Check sheet for the drawn part. Datum: minimum x, y, z corner. Units: mm. Coordinates: 2 decimals unless noted, no trailing zeros. Loops run counter-clockwise (first coordinate to the right, second up) from the corner with the lowest first, then second, coordinate; pieces in that order, holes last. Notation, with made-up numbers: (46.25, 24.5) - (63.25, 24.5) arc R13 ccw to (63.25, 40.5) - close; hole circle Ø1 at (70, -7). An arc over 180 degrees is marked (long way). Answer as CSV lines item,"result". Start each with the question number.
1. Cross-section at A-A (x = 6). Enter the section's corners in (y, z).
2. Material ranges on line 1 (X direction, y = 1, z = 35); line 2 (Y direction, x = 3, z = 30); line 3 (X direction, y = 3.2, z = 2), recorded low to high. Write a range as [from, to].
3. Cross-section at B-B (z = 30). Enter the section's corners in (x, y).
4. Cross-section at D-D (y = 2.5). State how many separate pieces and enclosed holes the cut face has, plus the area to 3 significant figures.
5. Gauge pin test, flat ends, axial feed: P1, Ø2, axis at y = 2.5, z = 10, coming from the +X side; P2, Ø2, axis at x = 10, y = 2.5, coming from the -Z side; P3, Ø0.8, axis at y = 2, z = 10.5, coming from the -X side. Record the tip position at first contact, or that the pin passes through.
6. Cross-section at C-C (x = 37). Enter the section's corners in (y, z), plus the area to 3 significant figures.
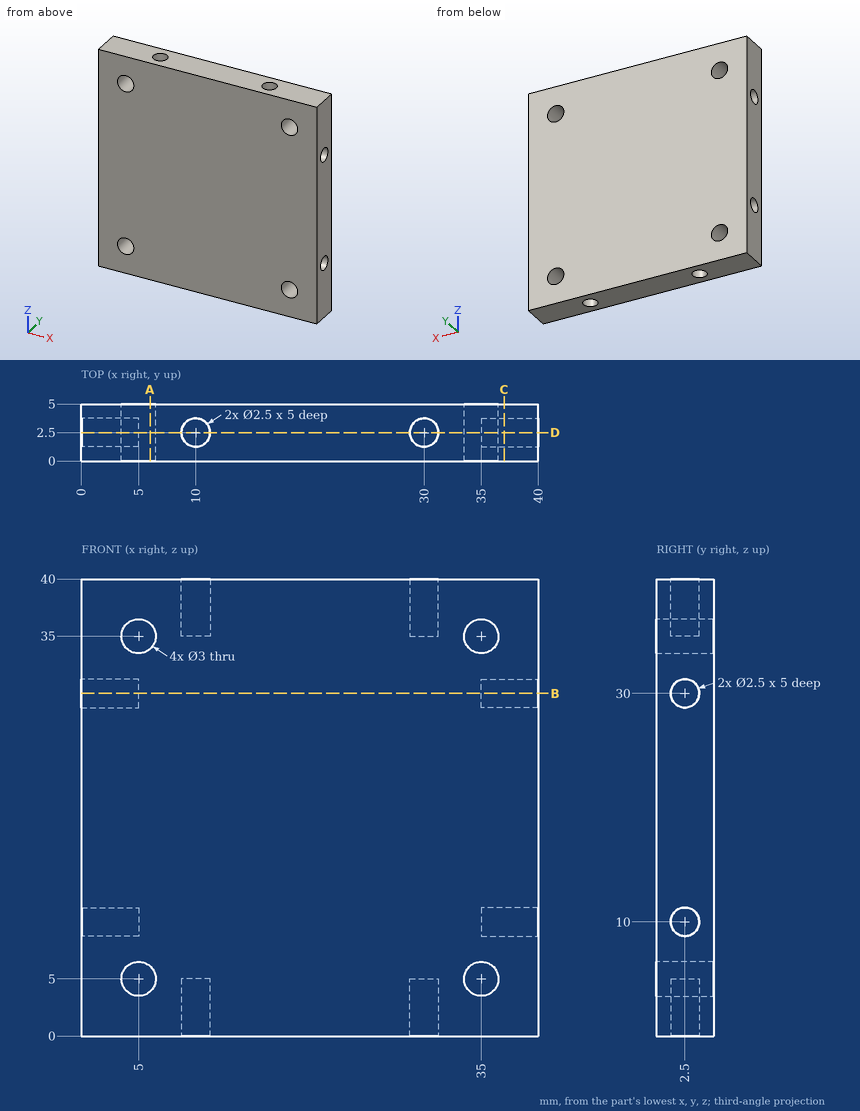
Values follow:
1,outline,"(0, 0) - (5, 0) - (5, 3.88) - (0, 3.88) - close; (0, 6.12) - (5, 6.12) - (5, 33.88) - (0, 33.88) - close; (0, 36.12) - (5, 36.12) - (5, 40) - (0, 40) - close"
2,line 1,"x = [0, 3.5], [6.5, 33.5], [36.5, 40]"
2,line 2,"y = [0, 1.25], [3.75, 5]"
2,line 3,"x = [0, 8.96], [11.04, 28.96], [31.04, 40]"
3,outline,"(0, 0) - (40, 0) - (40, 1.25) - (35, 1.25) - (35, 3.75) - (40, 3.75) - (40, 5) - (0, 5) - (0, 3.75) - (5, 3.75) - (5, 1.25) - (0, 1.25) - close"
4,separate pieces,"1"
4,enclosed holes,"4"
4,area,"1,470 mm²"
5,P1,"stops at x = 35"
5,P2,"stops at z = 5"
5,P3,"stops at x = 5"
6,outline,"(0, 0) - (5, 0) - (5, 40) - (0, 40) - close; hole circle Ø2.5 at (2.5, 10); hole circle Ø2.5 at (2.5, 30)"
6,area,"190 mm²"
